For this review, use the dimensioned drawing (mm, ordinates from the lowest corner) and the shaded views. Coordinates: 2 decimals unless noted, no trailing zeros. Order: outer loops, then holes, each group sorted by start corner. A loop starts at its lowest first (then second) coordinate and runs counter-clockwise, first axis right, second up. Notation, with made-up numbers: M -7.5,70 L 8.5,70 A29 cw 8.5,99 Z; hole C -14,-19.75 d5. An arc over 180 degrees is marked long. One line per item, written item: value.
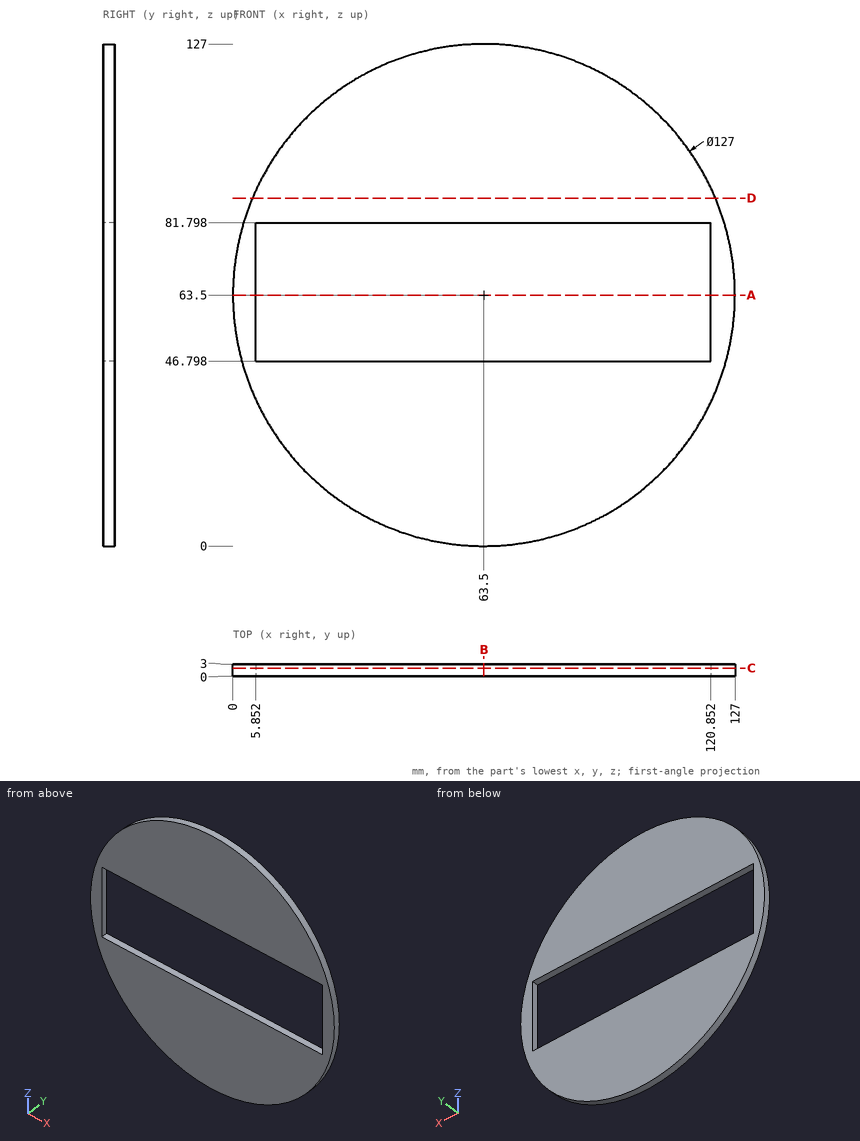
(1) We need section D-D, the plane z = 88. State the section outline as (x, y) points.
Geometry results:
outline: M 4.92,0 L 122.08,0 L 122.08,3 L 4.92,3 Z
(2) We need section C-C, the plane y = 2. State the section outline as (x, z) points, plus the area to 3 significant figures.
Geometry results:
outline: C 63.5,63.5 d127; hole M 5.85,46.8 L 120.85,46.8 L 120.85,81.8 L 5.85,81.8 Z
area: 8,640 mm2
(3) Insertion check: pin 1 Ø1.5 at (y, z) = (2.5, 85) entering from -X; pin 2 Ø0.9 at (y, z) = (1.5, 68) entering from -X; pin 3 Ø8 at (x, z) = (113, 73) entering from -Y; pin 4 Ø0.9 at (y, z) = (2, 57.5) entering from +X. Each pin has a flat end and moves straight along its axis. Give the tip position at first contact, or say it passes through.
Geometry results:
pin 1: stops at x = 3.49
pin 2: stops at x = 0.13
pin 3: passes through
pin 4: stops at x = 126.76
(4) For L1, parallel to Z at x = 63, y = 0.3; L2, parallel to X at y = 1.9, z = 65; L3, parallel to Z at x = 55.5, y = 1.2 (1 decimal), list the stretches that pass through material, from the lowest coordinate up.
Geometry results:
L1: z = 0 to 46.8, 81.8 to 127
L2: x = 0.02 to 5.85, 120.85 to 126.98
L3: z = 0.5 to 46.8, 81.8 to 126.5
(5) We need section B-B, the plane x = 63.5. State the section outline as (y, z) points, plus the area to 3 significant figures.
Geometry results:
outline: M 0,0 L 3,0 L 3,46.8 L 0,46.8 Z; M 0,81.8 L 3,81.8 L 3,127 L 0,127 Z
area: 276 mm2
(6) We need section A-A, the plane z = 63.5. State the section outline as (x, y) points.
Geometry results:
outline: M 0,0 L 5.85,0 L 5.85,3 L 0,3 Z; M 120.85,0 L 127,0 L 127,3 L 120.85,3 Z
